Check sheet for the modelled part. Datum: model origin and axes. Units: mm. Round coordinates to 2 decimals unless told otherwise and drop trailing zeros. Order: outer loops, then holes, each group sorted by start corner. A loop starts at its lowest first (then second) coordinate and runs counter-clockwise, first axis right, second up.
(1) Depth check by flat-ended pin: pin 1 (6 mm diameter, centred on x = -12.7, z = 38.1, fed in from -Y). Enter the tip coordinate at first touch or a pass-through.
(2) Sectioned sample at C-C, the plane y = 0.65. Enter the section's corners in (x, z).
(3) Sectioned sample at A-A, the plane x = -12.7. Enter the section's corners in (y, z) (1 decimal).
(4) Sectioned sample at B-B, the plane z = 38.1. Count the separate pieces of the cut face and the enclosed holes in it, and give its area (3 significant figures).
(5) Mould release check, pull along X, two halves, no side actions. Record for faces 1 (the flat face through (0, 2, 39)), 2 (the cylindrical face through (-77.17, 1.57, 41.19)), 3 (the flat face through (-47, 2, 0)), 4 (the flat face through (-95.25, 2, 38)): released by +X, released by -X, zero draft, split by the parting line, or undercut.
(6) Thickness scan on probe 1 along X at (y, z) = (1.5, 38.1); probe 2 along Z at (x, y) = (-12.7, 1.3); probe 3 along Z at (x, y) = (-11, 1.95). Record the ranges inside material, lowest first.
Autodesk Inventor part; units mm, degrees
ref_plane "YZ Plane" through (0, 0, 0) normal (1, 0, 0) x (0, 1, 0)
ref_plane "XZ Plane" through (0, 0, 0) normal (0, 1, 0) x (-1, 0, 0)
ref_plane "XY Plane" through (0, 0, 0) normal (0, 0, 1) x (1, 0, 0)
sketch "Sketch1" plane through (0, 0, 0) normal (0, 1, 0) x (-1, 0, 0)
  line L0 (0, 0) -> (95.25, 0)
  line L1 (95.25, 0) -> (95.25, 76.2)
  line L2 (95.25, 76.2) -> (0, 76.2)
  line L3 (0, 76.2) -> (0, 0)
  point P0 (76.2, 12.7)
  point P1 (12.7, 13.1017)
  point P2 (76.2, 38.1)
  point P3 (12.7, 38.1)
  dimension "d0" = 95.25
  dimension "d1" = 76.2
  dimension "d14" = 12.7
  dimension "d15" = 19.05
  dimension "d16" = 63.5
  dimension "d29" = 19.05
  dimension "d30" = 38.1
  dimension "d31" = 63.5
extrude "Extrusion2" add sketch "Sketch1" along normal blind 3.175
sketch "Sketch3" plane through (0, 3.175, 0) normal (0, 1, 0) x (1, 0, 0)
  line L0 (0, 0) -> (-95.25, 0)
  line L1 (-95.25, 0) -> (-95.25, -76.2)
  point P0 (-76.2, -12.7)
  point P1 (-12.7, -12.7)
  point P2 (-76.2, -38.1)
  point P3 (-12.7, -38.1)
  dimension "d19" = 19.05
  dimension "d20" = 12.7
  dimension "d21" = 63.5
  dimension "d32" = 25.4
  dimension "d33" = 63.5
  dimension "d34" = 19.05
hole "Hole3" at (-76.2, 3.175, 12.7) at (-12.7, 3.175, 12.7) at (-76.2, 3.175, 38.1) at (-12.7, 3.175, 38.1) direction (0, -1, 0) diameter 6.477 end through all
properties part number "slider"
Derived:
1. pin 1: passes through
2. outline: (-95.25, 0) - (0, 0) - (0, 76.2) - (-95.25, 76.2) - close; hole circle Ø6.48 at (-76.2, 12.7); hole circle Ø6.48 at (-76.2, 38.1); hole circle Ø6.48 at (-12.7, 12.7); hole circle Ø6.48 at (-12.7, 38.1)
3. outline: (0, 0) - (3.2, 0) - (3.2, 9.5) - (0, 9.5) - close; (0, 15.9) - (3.2, 15.9) - (3.2, 34.9) - (0, 34.9) - close; (0, 41.3) - (3.2, 41.3) - (3.2, 76.2) - (0, 76.2) - close
4. separate pieces: 3
4. enclosed holes: 0
4. area: 261 mm2
5. face 1: released by +X
5. face 2: undercut
5. face 3: zero draft
5. face 4: released by -X
6. probe 1: x = -95.25 to -79.44, -72.96 to -15.94, -9.46 to 0
6. probe 2: z = 0 to 9.46, 15.94 to 34.86, 41.34 to 76.2
6. probe 3: z = 0 to 9.94, 15.46 to 35.34, 40.86 to 76.2
